Source: three-view drawing plus pictorial views. Frame: mm from the lowest corner of the part. A direction names the side the tool comes from. Round coordinates to 2 decimals unless told otherwise and drop trailing zeros. Loops run counter-clockwise (first coordinate to the right, second up) from the corner with the lowest first, then second, coordinate; pieces in that order, holes last. Notation, with made-up numbers: (44, 78) -> (93, 78) arc R13 ccw to (93, 89) -> close; hole circle Ø4 at (19, 51). An arc over 180 degrees is marked (long way). Answer in a Markdown table with one row per item.
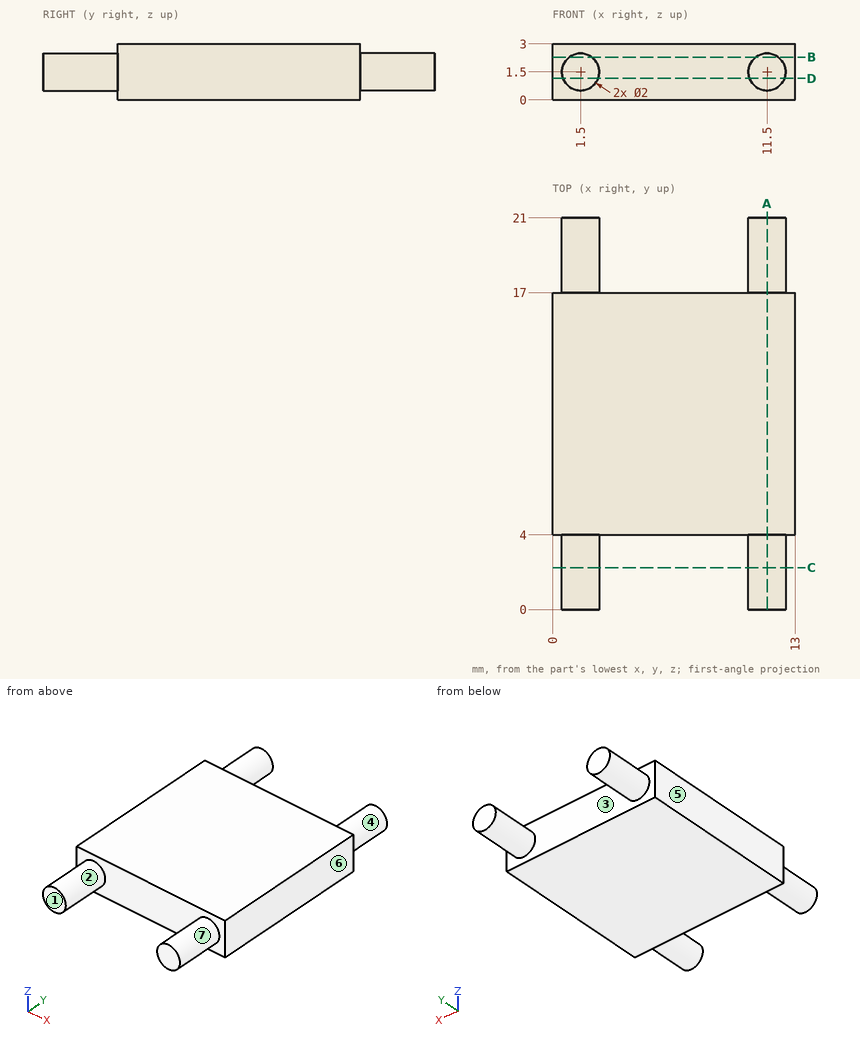
Item 1: Cut plane D-D (z = 1.15). Output: boundary loops of the cut face in (x, y), then the cut area to 3 significant figures.
Answer:
| item | result |
|---|---|
| outline | (0, 4) -> (0.56, 4) -> (0.56, 0) -> (2.44, 0) -> (2.44, 4) -> (10.56, 4) -> (10.56, 0) -> (12.44, 0) -> (12.44, 4) -> (13, 4) -> (13, 17) -> (12.44, 17) -> (12.44, 21) -> (10.56, 21) -> (10.56, 17) -> (2.44, 17) -> (2.44, 21) -> (0.56, 21) -> (0.56, 17) -> (0, 17) -> close |
| area | 199 mm² |
Item 2: Draft query along X for the marked faces 4, 5, 6 and 7. Return one class per face: pulls with the +X half, pulls with the -X half, needs draft (parallel to the pull), parting line crosses it, or undercut.
Answer:
| item | result |
|---|---|
| face 4 | undercut |
| face 5 | pulls with the -X half |
| face 6 | pulls with the +X half |
| face 7 | undercut |
Item 3: Reachability of the marked faces 1, 2 and 3 from +Z, -Z, +X, -X, +Y, -Y: full face, straight path, thin tool, end or side. Return the list, or none.
Answer:
| item | result |
|---|---|
| face 1 | +Z, -Z, +X, -X, -Y |
| face 2 | -Y |
| face 3 | +Y |
Item 4: Pin query (flat end, axial travel): pin 1 Ø1.5 at (x, y) = (11, 17) entering from -Z; pin 2 Ø1 at (x, z) = (7, 1) entering from -Y. Return the tip coordinate at first contact, or that it passes through.
Answer:
| item | result |
|---|---|
| pin 1 | stops at z = 0 |
| pin 2 | stops at y = 4 |
Item 5: Cut plane A-A (x = 11.5). Output: boundary loops of the cut face in (y, z).
Answer:
| item | result |
|---|---|
| outline | (0, 0.5) -> (4, 0.5) -> (4, 0) -> (17, 0) -> (17, 0.5) -> (21, 0.5) -> (21, 2.5) -> (17, 2.5) -> (17, 3) -> (4, 3) -> (4, 2.5) -> (0, 2.5) -> close |
Item 6: Cut plane C-C (y = 2.25). Output: boundary loops of the cut face in (x, z).
Answer:
| item | result |
|---|---|
| outline | circle Ø2 at (1.5, 1.5); circle Ø2 at (11.5, 1.5) |
Item 7: Line query: probe 1 along X at (y, z) = (2.75, 1.45); probe 2 along Y at (x, z) = (11, 0.3); probe 3 along X at (y, z) = (19, 0.9). Output: solid intervals per line, ascending. Write a range as [from, to].
Answer:
| item | result |
|---|---|
| probe 1 | x = [0.5, 2.5], [10.5, 12.5] |
| probe 2 | y = [4, 17] |
| probe 3 | x = [0.7, 2.3], [10.7, 12.3] |
Item 8: Cut plane B-B (z = 2.3). Output: boundary loops of the cut face in (x, y).
Answer:
| item | result |
|---|---|
| outline | (0, 4) -> (0.9, 4) -> (0.9, 0) -> (2.1, 0) -> (2.1, 4) -> (10.9, 4) -> (10.9, 0) -> (12.1, 0) -> (12.1, 4) -> (13, 4) -> (13, 17) -> (12.1, 17) -> (12.1, 21) -> (10.9, 21) -> (10.9, 17) -> (2.1, 17) -> (2.1, 21) -> (0.9, 21) -> (0.9, 17) -> (0, 17) -> close |
